```python
from build123d import *

# Parameters (mm, degrees)
SKETCH1_R           = 350
SKETCH1_R_2         = 100
BOSS_EXTRUDE1_DEPTH = 800
SKETCH2_W           = 250
SKETCH2_H           = 600
CUT_EXTRUDE1_DEPTH  = 25
SKETCH3_W           = 366
SKETCH3_H           = 400
CUT_EXTRUDE2_DEPTH  = 50


with BuildPart() as part:
    # Sketch1 → Boss-Extrude1 (new body)
    with BuildSketch(Plane(origin=(0, 0, 0), x_dir=(1, 0, 0), z_dir=(0, 1, 0))):
        Circle(SKETCH1_R)
        Circle(SKETCH1_R_2, mode=Mode.SUBTRACT)
    extrude(amount=BOSS_EXTRUDE1_DEPTH)

    # Sketch2 → Cut-Extrude1 (cut)
    with BuildSketch(Plane.XY.offset(350)):
        with Locations((5, 400)):
            Rectangle(SKETCH2_W, SKETCH2_H)
    extrude(amount=-CUT_EXTRUDE1_DEPTH, mode=Mode.SUBTRACT)

    # Sketch3 → Cut-Extrude2 (cut)
    with BuildSketch(Plane(origin=(350, 0, 0), x_dir=(0, 0, -1), z_dir=(1, 0, 0))):
        with Locations((-2.7, 400)):
            Rectangle(SKETCH3_W, SKETCH3_H)
    extrude(amount=-CUT_EXTRUDE2_DEPTH, mode=Mode.SUBTRACT)


solid = part.part
```
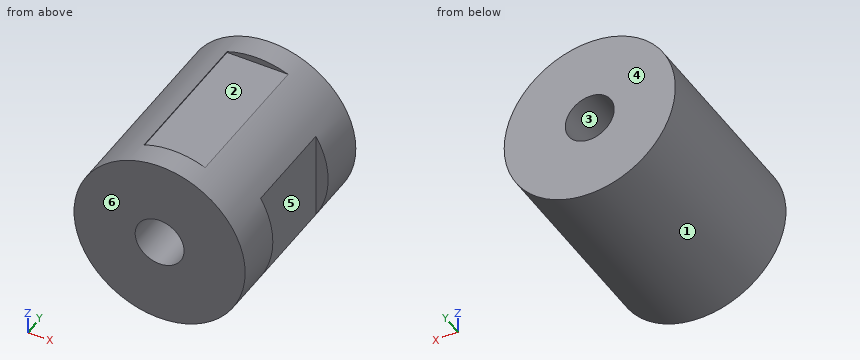
Check sheet for the modelled part. Datum: model origin and axes. Units: mm. Face numbers are marked on the shaded views. A direction names the side the tool comes from. Round coordinates to 2 decimals unless told otherwise and drop trailing zeros. Order: outer loops, then holes, each group sorted by start corner. A loop starts at its lowest first (then second) coordinate and runs counter-clockwise, first axis right, second up. Notation, with made-up numbers: (39.25, 52) -> (85.25, 52) arc R32 ccw to (85.25, 78) -> close; hole circle Ø6 at (3, 58.5). An arc over 180 degrees is marked (long way). Use CSV: the item, a comma, the result in double quotes.
(1) Tool access check on the marked faces 5 and 6. Record the directions out of +Z, -Z, +X, -X, +Y, -Y that give a thin tool (end or side, any length) a straight path to the whole face; none if there is none.
Worked out:
face 5,"+Z, -Z, +X"
face 6,"+Z, -Z, +X, -X, -Y"
(2) Depth check by flat-ended pin: pin 1 (6 mm diameter, centred on y = 376.5, z = -120.5, fed in from -X); pin 2 (6 mm diameter, centred on y = 665.5, z = -228, fed in from -X); pin 3 (3 mm diameter, centred on y = 437, z = 209, fed in from +X). Enter the tip coordinate at first touch or a pass-through.
Worked out:
pin 1,"x = -329.69"
pin 2,"x = -268.1"
pin 3,"x = 281.86"
(3) Cross-section at A-A (x = 0). Record the boundary of the cut face in (y, z), and give its area (3 significant figures).
Worked out:
outline,"(0, -350) -> (800, -350) -> (800, -100) -> (0, -100) -> close; (0, 100) -> (800, 100) -> (800, 350) -> (700, 350) -> (700, 325) -> (100, 325) -> (100, 350) -> (0, 350) -> close"
area,"385,000 mm²"
(4) Cross-section at C-C (y = 279.5). Record the boundary of the cut face in (x, z).
Worked out:
outline,"(-120, 325) -> (-120, 328.79) arc R350 ccw (long way) to (300, -180.28) -> (300, 180.28) arc R350 ccw to (129.9, 325) -> close; hole circle Ø200 at (0, 0)"
(5) Cross-section at D-D (x = 115). Record the boundary of the cut face in (y, z), and give its area (3 significant figures).
Worked out:
outline,"(0, -330.57) -> (800, -330.57) -> (800, 330.57) -> (700, 330.57) -> (700, 325) -> (100, 325) -> (100, 330.57) -> (0, 330.57) -> close"
area,"526,000 mm²"
(6) Draft check along Z on the marked faces 1, 2, 3 and 4. Enter one of: pulls with the +Z half, pulls with the -Z half, needs draft (parallel to the pull), parting line crosses it, or undercut.
Worked out:
face 1,"parting line crosses it"
face 2,"pulls with the +Z half"
face 3,"undercut"
face 4,"needs draft"
(7) Material ranges on line 1 along Z through (x, y) = (-5, 638.5); line 2 along Z through (x, y) = (0, 592); line 3 along X through (y, z) = (223, 0), recorded low to high. Write a range as from..to.
Worked out:
line 1,"-349.96..-99.87, 99.87..325"
line 2,"-350..-100, 100..325"
line 3,"-350..-100, 100..300"
(8) Cross-section at B-B (z = 0). Record the boundary of the cut face in (x, y), and give its area (3 significant figures).
Worked out:
outline,"(-350, 0) -> (-100, 0) -> (-100, 800) -> (-350, 800) -> close; (100, 0) -> (350, 0) -> (350, 200) -> (300, 200) -> (300, 600) -> (350, 600) -> (350, 800) -> (100, 800) -> close"
area,"380,000 mm²"
